Model file for the job. Use its own axes, mm. Give positions to 0.01 mm unless a question says otherwise; leave off trailing zeros. One line per item, written item: value. Start each with the question number.
(1) Drop flat-ended pins along their axis: P1, Ø4, axis at x = -123.5, z = 6, coming from the +Y side; P2, Ø4, axis at x = -69.5, y = -18, coming from the +Z side; P3, Ø6, axis at x = -191, y = -3, coming from the +Z side. Give the stop position or say it passes through.
(2) Probe L1, parallel to X at y = -5.75, z = 9.5; L2, parallel to X at y = -2.75, z = 13.75; L3, parallel to X at y = -11.75, z = 2.75. List the from-to ranges inside material, lowest first.
(3) Mould opens along Z. For faces 1 (the face through (-140.5, -3.01, 17.15)), 2 (the face through (-275.966, -9.86, 5.183)), 3 (the face through (-2, -10, 4)) say: pulls with the +Z half, pulls with the -Z half, needs draft (parallel to the pull), parting line crosses it, or undercut.
(4) Cut at B-B, the plane y = -16. State how many separate pieces and enclosed holes the cut face has, and give its area (3 significant figures).
from build123d import *

# Parameters (mm, degrees)
F0_W     = 285
F0_H     = 20
F1_DEPTH = 20
F2_R     = 9.99999
F3_R     = 5
F3_R_2   = 5.4133078472
F4_DEPTH = 20


# Not quite as in the source:
# - a fillet or chamfer is up to 0.001 mm smaller than in the source, because OpenCascade refuses the exact size


with BuildPart() as f1:
    # F0 (on Front) → F1 (new body)
    with BuildSketch(Plane.XZ):
        with Locations((-142.5, 10)):
            Rectangle(F0_W, F0_H)
    extrude(amount=F1_DEPTH)

    # F2 (radius 10 in the source; OpenCascade refuses exactly that, so slightly less here)
    f2_edges = [f1.edges().sort_by_distance(p)[0] for p in [
        (-142.5, -20, 20),
        (-142.5, 0, 20),
        (-142.5, -20, 0),
        (0, -10, 0),
        (-142.5, 0, 0),
        (-285, -10, 0),
        (0, -10, 20),
        (-285, -10, 20),
    ]]
    fillet(f2_edges, radius=F2_R)

    # F3 (on Front) → F4 (cut)
    with BuildSketch(Plane.XZ):
        with Locations((-274.8824357986, 10.0639369339)):
            Circle(F3_R)
        with Locations((-9.8824357986, 10.070726499)):
            Circle(F3_R_2)
    extrude(amount=F4_DEPTH, mode=Mode.SUBTRACT)


solid = f1.part
Answers follow:
1. P1: stops at y = -0.2
1. P2: stops at z = 18
1. P3: stops at z = 19.17
2. L1: x = -284.99 to -279.85, -269.91 to -15.27, -4.5 to -0.01
2. L2: x = -284.27 to -278.26, -271.5 to -13.85, -5.91 to -0.73
2. L3: x = -281.89 to -3.11
3. face 1: pulls with the +Z half
3. face 2: undercut
3. face 3: pulls with the -Z half
4. separate pieces: 1
4. enclosed holes: 2
4. area: 4,350 mm²
